Autodesk Inventor part; units mm, degrees
ref_plane "YZ Plane" through (0, 0, 0) normal (1, 0, 0) x (0, 1, 0)
ref_plane "XZ Plane" through (0, 0, 0) normal (0, 1, 0) x (-1, 0, 0)
ref_plane "XY Plane" through (0, 0, 0) normal (0, 0, 1) x (1, 0, 0)
sketch "Sketch2" plane through (0, 0, 0) normal (0, 0, 1) x (1, 0, 0)
  line L0 (-16.8, 0) -> (16.8, 0) construction
  line L1 (0, -21) -> (0, 21) construction
  line L2 (-12, -15) -> (12, -15)
  line L3 (12, -15) -> (12, 15)
  line L4 (12, 15) -> (-12, 15)
  line L5 (-12, 15) -> (-12, -15)
  circle A0 centre (7.02, 0) radius 1
  circle A1 centre (4.96389, 4.96389) radius 1
  circle A2 centre (0, 7.02) radius 1
  circle A3 centre (-4.96389, 4.96389) radius 1
  circle A4 centre (-7.02, 0) radius 1
  circle A5 centre (-4.96389, -4.96389) radius 1
  circle A6 centre (0, -7.02) radius 1
  circle A7 centre (4.96389, -4.96389) radius 1
  point P0 (0, 0)
  dimension "d3" = 30
  dimension "d4" = 24
  dimension "d5" = 7.02
  dimension "d6" = 2
  dimension "d9" = 360
extrude "Extrusion1" add sketch "Sketch2" along normal blind 3 contours L5 L4 L3 L2 | A0 | A1 | A2 | A3 | A4 | A5 | A6 | A7
sketch "Sketch1" plane through (0, 0, 0) normal (0, 1, 0) x (-1, 0, 0)
  line L0 (183.866798, 0) -> (-123.200788, 0) construction
  line L1 (-12, 0) -> (12, 0)
  line L2 (12, 0) -> (12, 3)
  line L3 (-12, 3) -> (12, 3)
  line L4 (-12, 0) -> (-12, 3)
  circle A0 centre (30, 12.361524) radius 10
  line L5 (-12, 0) -> (-12, 3)
  line L6 (25.615753, 21.349203) -> (-12, 3)
  line L7 (31.257448, 2.440898) -> (12, 0)
  circle A1 centre (30, 12.361524) radius 3
  dimension "d31" = 20
  dimension "d32" = 6
extrude "Extrusion6" add sketch "Sketch1" along normal blind 4 from surface at -15 contours L2 L3 L6 A0 L7 | A0 | A1
mirror "Mirror1" about plane through (0, 0, 0) normal (0, 1, 0) of "Extrusion6"
extrude "Extrusion7" cut sketch "Sketch2" along normal through all contours A0 | A1 | A2 | A3 | A4 | A5 | A6 | A7
extrude "Extrusion8" add sketch "Sketch1" along normal through all both and the other way through all contours A0 | A1
extrude "Extrusion9" cut sketch "Sketch1" along normal mid plane 9 contours A0 | A1
extrude "Extrusion10" cut sketch "Sketch1" along normal through all both and the other way through all contours A1
properties part number "bridge3"
Work out the finished part from the listing and answer in its coordinate system (mm). A direction names the side the tool comes from. Round coordinates to 2 decimals unless told otherwise and drop trailing zeros. Loops run counter-clockwise (first coordinate to the right, second up) from the corner with the lowest first, then second, coordinate; pieces in that order, holes last. Notation, with made-up numbers: (-8, 17.5) -> (31, 17.5) arc R6 ccw to (31, 27.5) -> close; hole circle Ø6 at (-22, -15.75). An arc over 180 degrees is marked (long way). Write each question's results on one line, items separated by ' | '. Start each with the question number.
1. Section A-A (y = 0) is taken. Determine the outline of the cut face in (x, z), plus the area to 3 significant figures.
2. Given pin 1 Ø2.5 at (x, y) = (-4.96, -4.96) entering from +Z; pin 2 Ø3.5 at (y, z) = (-4.5, 2) entering from -X; pin 3 Ø4 at (y, z) = (-7, 7) entering from -X; pin 4 Ø4 at (y, z) = (-5, 10.5) entering from -X, each flat-ended and moving along its own axis, determine where each tip first touches the part or whether it passes through.
3. A tool of negligible diameter and unlimited length cuts with its end or side. For faces 3 (the face through (-12, 0, 1)), 4 (the face through (-6.545, 13.028, 12.046)), from which of +Z, -Z, +X, -X, +Y, -Y can it reach the whole face along a straight path? Write none if from no direction.
4. Section D-D (y = 9.5) is taken. Determine the outline of the cut face in (x, z).
5. Section C-C (x = -29.5) is taken. Determine the outline of the cut face in (y, z).
6. Find the intervals of material crossed by probe 1 along Y at (x, z) = (-23, 12.5); probe 2 along Y at (x, z) = (4.5, 2.5); probe 3 along X at (y, z) = (7.02, 1.7), in increasing order. Write a range as from..to.
7. For a pull along Y with two mould halves and no side action, classify faces 1 (the face through (-21.494, 13.028, 1.203)), 2 (the face through (0, 0, 3)) as +Y half, -Y half, draft (parallel to the pull), parting line (faces both ways), or undercut.
8. Section B-B (y = -7.02) is taken. Determine the outline of the cut face in (x, z).
Evaluation:
1) outline: (-12, 0) -> (-8.02, 0) -> (-8.02, 3) -> (-12, 3) -> close; (-6.02, 0) -> (6.02, 0) -> (6.02, 3) -> (-6.02, 3) -> close; (8.02, 0) -> (12, 0) -> (12, 3) -> (8.02, 3) -> close | area: 60.0 mm2
2) pin 1: stops at z = 3 | pin 2: stops at x = -35.08 | pin 3: stops at x = -39.42 | pin 4: stops at x = -40
3) face 3: +Z, -Z | face 4: +Z, +X, +Y, -Y
4) outline: circle Ø20 at (-30, 12.36); (-12, 0) -> (12, 0) -> (12, 3) -> (-12, 3) -> close; hole circle Ø6 at (-30, 12.36)
5) outline: (-15, 2.22) -> (-11, 2.22) -> (-11, 2.37) -> (-4.5, 2.37) -> (-4.5, 9.4) -> (-15, 9.4) -> close; (-15, 15.32) -> (-4.5, 15.32) -> (-4.5, 22.35) -> (-15, 22.35) -> close; (4.5, 2.37) -> (11, 2.37) -> (11, 2.22) -> (15, 2.22) -> (15, 9.4) -> (4.5, 9.4) -> close; (4.5, 15.32) -> (15, 15.32) -> (15, 22.35) -> (4.5, 22.35) -> close
6) probe 1: y = -15..-4.5, 4.5..15 | probe 2: y = -15..-5.85, -4.08..4.08, 5.85..15 | probe 3: x = -12..-1, 1..12
7) face 1: draft | face 2: undercut
8) outline: circle Ø20 at (-30, 12.36); (-12, 0) -> (-1, 0) -> (-1, 3) -> (-12, 3) -> close; (1, 0) -> (12, 0) -> (12, 3) -> (1, 3) -> close; hole circle Ø6 at (-30, 12.36)
